Design review of the part built by this model. Coordinates are the model's own, in mm. Face numbers are marked on the shaded views. A direction names the side the tool comes from. Give positions to 0.01 mm unless a question says otherwise; leave off trailing zeros. Order: outer loops, then holes, each group sorted by start corner. A loop starts at its lowest first (then second) coordinate and runs counter-clockwise, first axis right, second up. Notation, with made-up numbers: (50, 54) -> (80, 54) arc R11 ccw to (80, 67) -> close; hole circle Ø9 at (-24.5, 17.5). An arc over 180 degrees is marked (long way). Return JSON: item names as keys, results as strings.
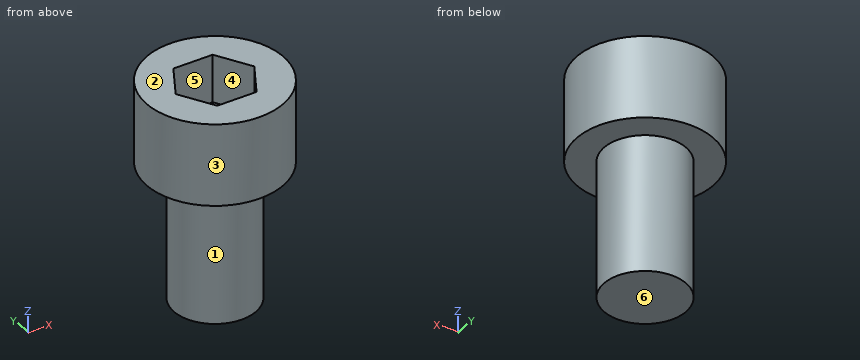
```python
from build123d import *

# Parameters (mm, degrees)
CUT_EXTRUDE1_DEPTH = 3.5


with BuildPart() as part:
    # Sketch1 → Revolve1 (revolve)
    with BuildSketch(Plane(origin=(0, 0, 0), x_dir=(0, 0, -1), z_dir=(1, 0, 0)), mode=Mode.PRIVATE) as revolve1_sk:
        Polygon((-6, 0), (-6, 5), (0, 5), (0, 3), (10, 3), (10, 0), align=None)
    revolve(revolve1_sk.sketch.rotate(Axis((0, 0, 5.584882278), (0, 0, -1)), 180), axis=Axis((0, 0, 5.584882278), (0, 0, -1)))

    # Sketch2 → Cut-Extrude1 (cut)
    with BuildSketch(Plane.XY.offset(6)):
        Polygon((1.443375673, -2.5), (2.886751346, 0), (1.443375673, 2.5), (-1.443375673, 2.5), (-2.886751346, 0), (-1.443375673, -2.5), align=None)
    extrude(amount=-CUT_EXTRUDE1_DEPTH, mode=Mode.SUBTRACT)


solid = part.part
```
Item 1: Machinability: for the marked faces 1 and 2, which of the approach directions +Z, -Z, +X, -X, +Y, -Y give a long, thin tool a straight path to every point of the face, cutting with its end or side? Answer none if there is none.
Result set:
{"face 1": "-Z", "face 2": "+Z, +X, -X, +Y, -Y"}
Item 2: Add section A-A (x = -1.75). Give the boundary of the cut face in (y, z), plus the area to 3 significant figures.
Result set:
{"outline": "(-4.68, 0) -> (-2.44, 0) -> (-2.44, -10) -> (2.44, -10) -> (2.44, 0) -> (4.68, 0) -> (4.68, 6) -> (1.97, 6) -> (1.97, 2.5) -> (-1.97, 2.5) -> (-1.97, 6) -> (-4.68, 6) -> close", "area": "91.2 mm^2"}
Item 3: For pin 1 (3 mm diameter, centred on y = -2.5, z = -8, fed in from +X); pin 2 (5 mm diameter, centred on y = 3.5, z = 3.5, fed in from +X); pin 3 (1.5 mm diameter, centred on x = 0.5, y = -0.5, fed in from +Z), all flat-tipped, find the tip position at first contact; note any pin that passes through.
Result set:
{"pin 1": "stops at x = 2.83", "pin 2": "stops at x = 4.9", "pin 3": "stops at z = 2.5"}
Item 4: Add section C-C (z = 1.75). Give the boundary of the cut face in (x, y), plus the area to 3 significant figures.
Result set:
{"outline": "circle Ø10 at (0, 0)", "area": "78.5 mm^2"}
Item 5: Wall thickness on L1, parallel to Z at x = 4.25, y = -0.5; L2, parallel to Z at x = -0.25, y = 1; L3, parallel to X at y = 1, z = 4: over which ranges is each line inside the solid? List them lowest first. Write a range as [from, to].
Result set:
{"L1": "z = [0, 6]", "L2": "z = [-10, 2.5]", "L3": "x = [-4.9, -2.31], [2.31, 4.9]"}
Item 6: Add section D-D (y = -3.25). Give the boundary of the cut face in (x, z), plus the area to 3 significant figures.
Result set:
{"outline": "(-3.8, 0) -> (3.8, 0) -> (3.8, 6) -> (-3.8, 6) -> close", "area": "45.6 mm^2"}
Item 7: Add section B-B (y = -2). Give the boundary of the cut face in (x, z), plus the area to 3 significant figures.
Result set:
{"outline": "(-4.58, 0) -> (-2.24, 0) -> (-2.24, -10) -> (2.24, -10) -> (2.24, 0) -> (4.58, 0) -> (4.58, 6) -> (1.73, 6) -> (1.73, 2.5) -> (-1.73, 2.5) -> (-1.73, 6) -> (-4.58, 6) -> close", "area": "87.6 mm^2"}
Item 8: Mouldability with a two-part tool opening along Y and no side actions: class the marked faces 3, 4, 5 and 6 as released by +Y, released by -Y, zero draft, split by the parting line, or undercut.
Result set:
{"face 3": "split by the parting line", "face 4": "undercut", "face 5": "undercut", "face 6": "zero draft"}
